CAD build for the part. Positions are in the model's coordinates, mm. A direction names the side the tool comes from. Give positions to 0.01 mm unless a question says otherwise; leave off trailing zeros. Write each loop counter-clockwise with the first axis right and the second up, starting at its lowest first coordinate (ties: lowest second). Pieces come first, ordered by that corner, then holes. Notation, with made-up numbers: (29.25, 39.5) - (51.25, 39.5) arc R28 cw to (51.25, 59.5) - close; hole circle Ø11 at (24, 35). An arc over 180 degrees is marked (long way). Answer as a JSON object with one key per item and string values.
from build123d import *

# Parameters (mm, degrees)
F0_W     = 180.622216
F0_H     = 140.405509
F0_W_2   = 194.250329
F0_H_2   = 195.742518
F0_W_3   = 200.377738
F0_H_3   = 113.020826
F1_DEPTH = 203.2
F2_W     = 74.582949
F2_H     = 85.822828
F3_DEPTH = 12.7
F4_W     = 134.511486
F4_H     = 63.10866
F5_DEPTH = 6.35
F6_W     = 128.129702
F6_H     = 63.10866
F7_DEPTH = 6.35


with BuildPart() as f1:
    # F0 (on Top) → F1 (new body)
    with BuildSketch(Plane.XY):
        with Locations((-436.033275, -70.202754)):
            Rectangle(F0_W, F0_H)
        Polygon((-151.471838, 0), (-345.722167, 0), (-345.722167, -140.405509), (-304.799954, -140.405509), (-304.799954, -178.505509), (-150.988865, -178.505509), (-150.988865, -140.405509), (0, -140.405509), (0, 0), (200.377738, 0), (200.377738, 178.373605), (0, 178.373605), (0, 291.394431), (-345.722167, 291.394431), (-345.722167, 195.742518), (-151.471838, 195.742518), align=None)
        with Locations((-248.597002, 97.871259)):
            Rectangle(F0_W_2, F0_H_2)
        with Locations((100.188869, 234.884018)):
            Rectangle(F0_W_3, F0_H_3)
        with Locations((100.188869, -70.202754)):
            Rectangle(F0_W_3, F0_H)
    extrude(amount=F1_DEPTH)

    # F2 (on face) → F3 (cut)
    with BuildSketch(Plane.XZ.offset(178.505509)):
        with Locations((-236.978226, 42.911414)):
            Rectangle(F2_W, F2_H)
    extrude(amount=-F3_DEPTH, mode=Mode.SUBTRACT)

    # F4 (on face) → F5 (cut)
    with BuildSketch(Plane.XZ.offset(140.405509)):
        with Locations((-67.255743, 132.67624)):
            Rectangle(F4_W, F4_H)
    extrude(amount=-F5_DEPTH, mode=Mode.SUBTRACT)

    # F6 (on face) → F7 (cut)
    with BuildSketch(Plane.XZ.offset(140.405509)):
        with Locations((110.273594, 132.67624)):
            Rectangle(F6_W, F6_H)
    extrude(amount=-F7_DEPTH, mode=Mode.SUBTRACT)


solid = f1.part
(1) 3-axis set-ups, long thin cutter, end or side, ignore diameter. For faces 1 (the face through (109, -134.056, 133)), 2 (the face through (99, -140.406, 100)), 3 (the face through (-345.722, 97, 100)), 4 (the face through (-304.8, -159, 100)): which of +Z, -Z, +X, -X, +Y, -Y reach the whole face in a straight line?
Answer key:
{"face 1": "-Y", "face 2": "+Z, -Z, +X, -Y", "face 3": "+Z, -Z, -X, +Y", "face 4": "+Z, -Z, -X, -Y"}
(2) Saw through at B-B, the plane x = -83. Give the cut face in (y, z), and give its area (3 significant figures).
Answer key:
{"outline": "(-140.41, 0) - (291.39, 0) - (291.39, 203.2) - (-140.41, 203.2) - (-140.41, 164.23) - (-134.06, 164.23) - (-134.06, 101.12) - (-140.41, 101.12) - close", "area": "87,300 mm²"}
(3) Pull direction Z, two halves, no side cores. Call faces 5 (the face through (-68, -134.056, 133)), 6 (the face through (-150.989, -160, 100)), 7 (the face through (-87, 60, 203.2)): pulls with the +Z half, pulls with the -Z half, needs draft (parallel to the pull), parting line crosses it, or undercut.
Answer key:
{"face 5": "undercut", "face 6": "needs draft", "face 7": "pulls with the +Z half"}
(4) Probe L1, parallel to Y at x = -69, z = 28.5; L2, parallel to Y at x = -485.5, z = 15; L3, parallel to X at y = 251.5, z = 12. List the from-to ranges inside material, lowest first. Write a range as [from, to].
Answer key:
{"L1": "y = [-140.41, 291.39]", "L2": "y = [-140.41, 0]", "L3": "x = [-345.72, 200.38]"}
(5) Saw through at D-D, the plane y = 124. Give the cut face in (x, z), and give its area (3 significant figures).
Answer key:
{"outline": "(-345.72, 0) - (200.38, 0) - (200.38, 203.2) - (-345.72, 203.2) - close", "area": "111,000 mm²"}
(6) Flat gauge pins, fed straight in: P1, Ø19, axis at y = -161.5, z = 141, coming from the -X side; P2, Ø12.5, axis at x = -321.5, z = 112, coming from the -Y side; P3, Ø10, axis at y = -170, z = 59.5, coming from the +X side. Where does each tip first touch, or does it go through?
Answer key:
{"P1": "stops at x = -304.8", "P2": "stops at y = -140.41", "P3": "stops at x = -150.99"}
(7) Saw through at C-C, the plane z = 22.5. Give the cut face in (x, y).
Answer key:
{"outline": "(-526.34, -140.41) - (-304.8, -140.41) - (-304.8, -178.51) - (-274.27, -178.51) - (-274.27, -165.81) - (-199.69, -165.81) - (-199.69, -178.51) - (-150.99, -178.51) - (-150.99, -140.41) - (200.38, -140.41) - (200.38, 291.39) - (-345.72, 291.39) - (-345.72, 0) - (-526.34, 0) - close"}
(8) Saw through at A-A, the plane z = 138.5. Give the cut face in (x, y), and give its area (3 significant figures).
Answer key:
{"outline": "(-526.34, -140.41) - (-304.8, -140.41) - (-304.8, -178.51) - (-150.99, -178.51) - (-150.99, -140.41) - (-134.51, -140.41) - (-134.51, -134.06) - (0, -134.06) - (0, -140.41) - (46.21, -140.41) - (46.21, -134.06) - (174.34, -134.06) - (174.34, -140.41) - (200.38, -140.41) - (200.38, 291.39) - (-345.72, 291.39) - (-345.72, 0) - (-526.34, 0) - close", "area": "265,000 mm²"}
